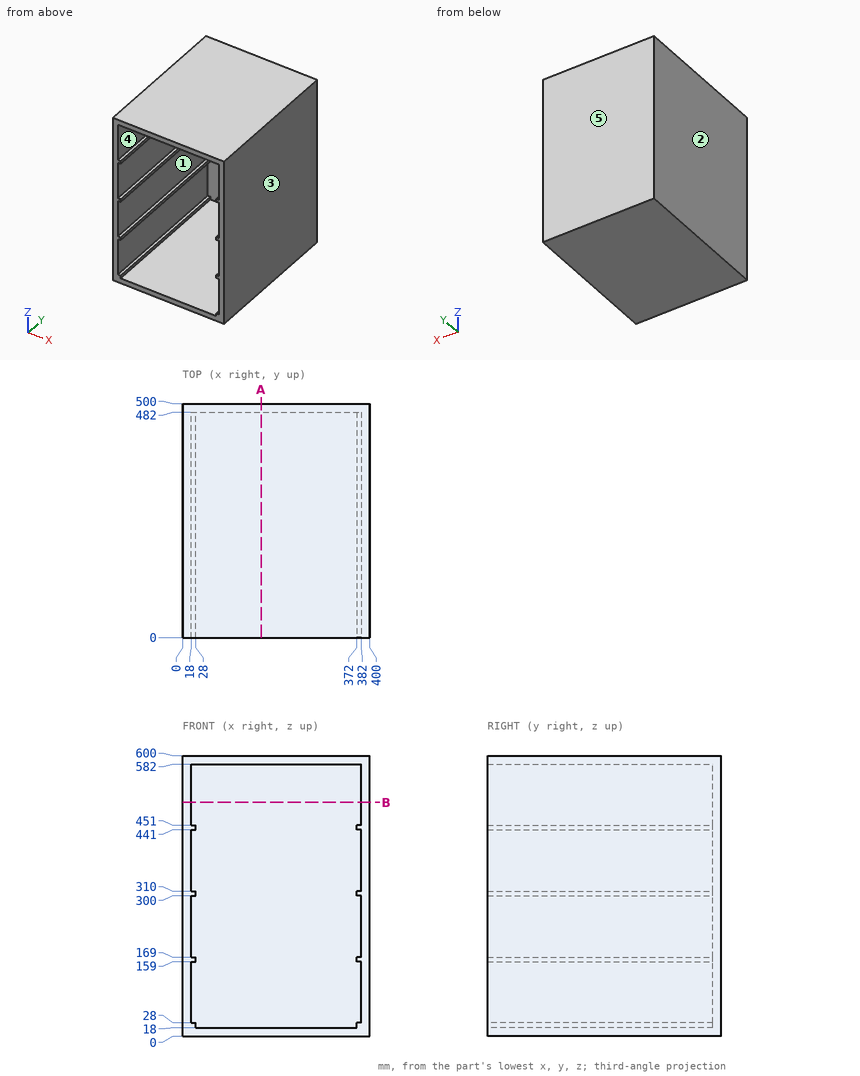
Design review of the part shown in the three views and the two pictorial views. Dimensions are in mm from the part's minimum x, y and z. A direction names the side the tool comes from. Give positions to 0.01 mm unless a question says otherwise; leave off trailing zeros. Loops run counter-clockwise (first coordinate to the right, second up) from the corner with the lowest first, then second, coordinate; pieces in that order, holes last. Notation, with made-up numbers: (82, 69) - (127, 69) arc R34 cw to (127, 105) - close; hole circle Ø9 at (32.5, -27). An arc over 180 degrees is marked (long way). Answer as a JSON object with one key per item and string values.
Q1. Add section B-B on z = 500. State the section outline as (x, y) points.
Worked out:
{"outline": "(0, 0) - (18, 0) - (18, 482) - (382, 482) - (382, 0) - (400, 0) - (400, 500) - (0, 500) - close"}
Q2. Mouldability with a two-part tool opening along X and no side actions: class the marked faces 3, 4 and 5 as +X half, -X half, draft (parallel to the pull), parting line (faces both ways), or undercut.
Worked out:
{"face 3": "+X half", "face 4": "undercut", "face 5": "draft"}
Q3. To check wall thickness, follow line 1 along Z through (x, y) = (256.5, 268); line 2 along Z through (x, y) = (20.5, 321.5); line 3 along X through (y, z) = (147.5, 364.5). State the ranges of each line that lie inside material, in increasing order.
Worked out:
{"line 1": "z = 0 to 18, 582 to 600", "line 2": "z = 0 to 28, 159 to 169, 300 to 310, 441 to 451, 582 to 600", "line 3": "x = 0 to 18, 382 to 400"}
Q4. For the marked faces 1 and 2, list the 3-axis set-ups (+Z, -Z, +X, -X, +Y, -Y) from which the entire face can be reached by the end or side of a thin tool; tool diameter is ignored.
Worked out:
{"face 1": "-Y", "face 2": "+Z, -Z, -X, +Y, -Y"}
Q5. Add section A-A on x = 168. State the section outline as (y, z) points, plus the area to 3 significant figures.
Worked out:
{"outline": "(0, 0) - (500, 0) - (500, 600) - (0, 600) - (0, 582) - (482, 582) - (482, 18) - (0, 18) - close", "area": "28,200 mm^2"}
Q6. Insertion check: pin 1 (4 mm diameter, centred on x = 280, z = 388.5, fed in from -Y). The pin has a flat end and moves straight along its axis. Give the tip position at first contact, or say it passes through.
Worked out:
{"pin 1": "stops at y = 482"}
